```python
from build123d import *

# Parameters (mm, degrees)
F0_R     = 4.167188
F0_W     = 17.78
F0_H     = 15.24
F1_DEPTH = 3.175


with BuildPart() as f1:
    # F0 (on Top) → F1 (new body)
    with BuildSketch(Plane.XY):
        with BuildLine():
            Line((25.4, 25.671175), (25.4, 0.271175))
            Line((25.4, 0.271175), (50.8, 0.271175))
            Line((50.8, 0.271175), (50.8, 25.671175))
            Line((50.8, 25.671175), (177.8, 25.671175))
            Line((177.8, 25.671175), (304.8, 25.671175))
            Line((304.8, 25.671175), (304.8, 0.271175))
            Line((304.8, 0.271175), (330.2, 0.271175))
            Line((330.2, 0.271175), (330.2, 25.671175))
            Line((330.2, 25.671175), (355.6, 25.671175))
            Line((355.6, 25.671175), (355.6, 46.595866))
            ThreePointArc((355.6, 46.595866), (342.881064, 48.726049), (330.2, 51.071175))
            Line((330.2, 51.071175), (304.8, 51.071175))
            ThreePointArc((304.8, 51.071175), (241.572069, 41.922444), (177.8, 38.102263))
            ThreePointArc((177.8, 38.102263), (114.027931, 41.922444), (50.8, 51.071175))
            Line((50.8, 51.071175), (25.4, 51.071175))
            ThreePointArc((25.4, 51.071175), (12.718936, 48.726049), (0, 46.595866))
            Line((0, 46.595866), (0, 25.671175))
            Line((0, 25.671175), (25.4, 25.671175))
        make_face()
        with Locations((38.1, 12.971175)):
            Circle(F0_R, mode=Mode.SUBTRACT)
        with Locations((317.5, 12.971175)):
            Circle(F0_R, mode=Mode.SUBTRACT)
        with Locations((12.7, 37.101175)):
            Rectangle(F0_W, F0_H, mode=Mode.SUBTRACT)
        with BuildLine():
            ThreePointArc((31.115, 46.308675), (30.32125, 47.102425), (31.115, 47.896175))
            Line((31.115, 47.896175), (45.085, 47.896175))
            ThreePointArc((45.085, 47.896175), (45.87875, 47.102425), (45.085, 46.308675))
            Line((45.085, 46.308675), (31.115, 46.308675))
        make_face(mode=Mode.SUBTRACT)
        with Locations((342.9, 37.101175)):
            Rectangle(F0_W, F0_H, mode=Mode.SUBTRACT)
        with BuildLine():
            Line((310.515, 47.896175), (324.485, 47.896175))
            ThreePointArc((324.485, 47.896175), (325.27875, 47.102425), (324.485, 46.308675))
            Line((324.485, 46.308675), (310.515, 46.308675))
            ThreePointArc((310.515, 46.308675), (309.72125, 47.102425), (310.515, 47.896175))
        make_face(mode=Mode.SUBTRACT)
    extrude(amount=F1_DEPTH)


solid = f1.part
```
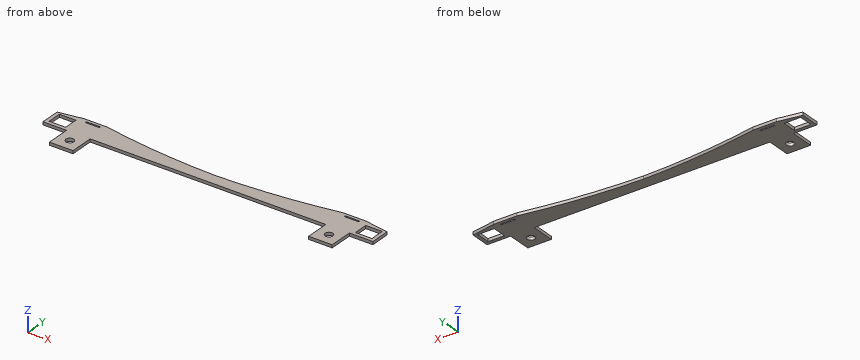
Model file for the job. Use its own axes, mm. Give positions to 0.01 mm unless a question says otherwise; leave off trailing zeros. Write each loop counter-clockwise with the first axis right and the second up, starting at its lowest first coordinate (ties: lowest second). Pieces come first, ordered by that corner, then holes. Notation, with made-up numbers: (36, 11.5) -> (69, 11.5) arc R33 ccw to (69, 48.5) -> close; hole circle Ø6 at (67, -27.5). An arc over 180 degrees is marked (long way). Use CSV: the item, a comma, the result in double quotes. Start each with the question number.
1) Cut at C-C on z = 1.9. Count the separate pieces of the cut face and the enclosed holes in it, plus the area to 3 significant figures.
2) Drill centre lines: L1, parallel to X at y = 36, z = 0.2; L2, parallel to Y at x = 38.1, z = 1.6; L3, parallel to X at y = 5, z = 0.25. Where is each one in solid material? Low to high.
3) Cut at B-B on y = 35. List the corners of the cut face in (x, z) (3 decimals), plus the area to 3 significant figures.
4) Cut at D-D on x = 265. List the corners of the cut face in (y, z) (3 decimals), plus the area to 3 significant figures.
5) Cut at A-A on x = 317.5. List the corners of the cut face in (y, z) (3 decimals), plus the area to 3 significant figures.
6) Pin check, flat tips, straight feed: P1, Ø1.5, axis at x = 120, z = 2, coming from the -Y side; P2, Ø1.6, axis at y = 17, z = 2, coming from the +X side. Stop position of each tip, or through.
Final values:
1,separate pieces,"1"
1,enclosed holes,"6"
1,area,"7,400 mm2"
2,L1,"x = 0 to 3.81, 21.59 to 334.01, 351.79 to 355.6"
2,L2,"y = 0.27 to 8.8, 17.14 to 46.31, 47.9 to 51.07"
2,L3,"x = 25.4 to 50.8, 304.8 to 330.2"
3,outline,"(0, 0) -> (3.81, 0) -> (3.81, 3.175) -> (0, 3.175) -> close; (21.59, 0) -> (334.01, 0) -> (334.01, 3.175) -> (21.59, 3.175) -> close; (351.79, 0) -> (355.6, 0) -> (355.6, 3.175) -> (351.79, 3.175) -> close"
3,area,"1,020 mm2"
4,outline,"(25.671, 0) -> (44.682, 0) -> (44.682, 3.175) -> (25.671, 3.175) -> close"
4,area,"60.4 mm2"
5,outline,"(0.271, 0) -> (8.804, 0) -> (8.804, 3.175) -> (0.271, 3.175) -> close; (17.138, 0) -> (46.309, 0) -> (46.309, 3.175) -> (17.138, 3.175) -> close; (47.896, 0) -> (51.071, 0) -> (51.071, 3.175) -> (47.896, 3.175) -> close"
5,area,"130 mm2"
6,P1,"stops at y = 25.67"
6,P2,"stops at x = 330.2"
